Autodesk Inventor part; units mm, degrees
ref_plane "YZ Plane" through (0, 0, 0) normal (1, 0, 0) x (0, 1, 0)
ref_plane "XZ Plane" through (0, 0, 0) normal (0, 1, 0) x (-1, 0, 0)
ref_plane "XY Plane" through (0, 0, 0) normal (0, 0, 1) x (1, 0, 0)
sketch "Sketch1" plane through (0, 0, 0) normal (0, 0, 1) x (1, 0, 0)
  circle A0 centre (0, 0) radius 38.1
  line L0 (7.852, 0) -> (3.926, -6.8)
  line L1 (3.926, -6.8) -> (-3.926, -6.8)
  line L2 (-3.926, -6.8) -> (-7.852, 0)
  line L3 (-7.852, 0) -> (-3.926, 6.8)
  line L4 (-3.926, 6.8) -> (3.926, 6.8)
  line L5 (3.926, 6.8) -> (7.852, 0)
  circle A1 centre (0, 0) radius 31.75 construction
  circle A2 centre (0, 31.75) radius 2.413
  circle A3 centre (-15.875, 27.4963) radius 2.413
  circle A4 centre (-27.4963, 15.875) radius 2.413
  circle A5 centre (-31.75, 0) radius 2.413
  circle A6 centre (-27.4963, -15.875) radius 2.413
  circle A7 centre (-15.875, -27.4963) radius 2.413
  circle A8 centre (0, -31.75) radius 2.413
  circle A9 centre (15.875, -27.4963) radius 2.413
  circle A10 centre (27.4963, -15.875) radius 2.413
  circle A11 centre (31.75, 0) radius 2.413
  circle A12 centre (27.4963, 15.875) radius 2.413
  circle A13 centre (15.875, 27.4963) radius 2.413
  line L6 (-9.525, 25.4) -> (-3.9688, 13.15)
  line L7 (-3.9688, 13.15) -> (3.9688, 13.15)
  line L8 (3.9688, 13.15) -> (9.525, 25.4)
  line L9 (9.525, 25.4) -> (-9.525, 25.4)
  line L10 (0, -53.34) -> (0, 53.34) construction
  circle A14 centre (0, 0) radius 25.4 construction
  line L11 (0, 29.337) -> (0, 25.4)
  line L12 (0, 38.1) -> (0, 25.4)
  dimension "d0" = 76.2
  dimension "d2" = 63.5
  dimension "d3" = 4.826
  dimension "d1" = 13.6
  dimension "d6" = 360
  dimension "d16" = 6.35
  dimension "d18" = 7.9375
  dimension "d19" = 19.05
  dimension "d20" = 12.7
extrude "Extrusion1" add sketch "Sketch1" along normal blind 3.175 contours L9 L8 L7 L6 | A0
extrude "Extrusion2" cut sketch "Sketch1" along normal blind 3.175 contours L9 L8 L7 L6
fillet "Fillet1" radius 3.175 4 edges at (-9.525, 25.4, 1.5875) (9.525, 25.4, 1.5875) (-3.9688, 13.15, 1.5875) (3.9688, 13.15, 1.5875)
pattern_circular "Circular Pattern1" count 6 over 360 about axis through (0, 0, 0) along (0, 0, 1) of "Extrusion2", "Fillet1"
properties part number "ThickWheelPlate_v83DPrintable" material "Steel, Alloy"
The listing builds one solid part. Answer for the finished solid, in the listing's coordinates (mm). Round coordinates to 2 decimals unless told otherwise and drop trailing zeros. Order: outer loops, then holes, each group sorted by start corner. A loop starts at its lowest first (then second) coordinate and runs counter-clockwise, first axis right, second up. Notation, with made-up numbers: M 13.25,53 L 44.25,53 A20 cw 44.25,86 Z; hole C 89,-26.5 d9. An arc over 180 degrees is marked long. Answer in a Markdown table with one row per item. Add a question column.
1) The part is cut by section A-A on x = 0. Determine the outline of the cut face in (y, z) (3 decimals).
2) The part is cut by section D-D on y = -1. Determine the outline of the cut face in (x, z) (3 decimals).
3) The part is cut by section B-B on y = 31.75. Determine the outline of the cut face in (x, z) (3 decimals), plus the area to 3 significant figures.
4) Consider line 1 along Y through (x, z) = (0, 0.7); line 2 along Y through (x, z) = (-1.5, 0.85); line 3 along Y through (x, z) = (15, 1.2). Determine where each line is inside the solid, lowest interval first. Write a range as from..to.
5) Determine the mould class of faces 1 (the face through (-29.448, -0.725, 1.565)), 2 (the face through (-30.235, 23.183, 1.565)), 3 (the face through (13.671, -3.662, 1.61)) for opening direction Y: pulls with the +Y half, pulls with the -Y half, needs draft (parallel to the pull), parting line crosses it, or undercut.
6) Flat-ended cylindrical pins translate along their axes: pin 1 Ø1.6 at (x, z) = (-0.5, 1.5) entering from +Y; pin 2 Ø1.5 at (y, z) = (-8, 1) entering from +X. Find the tip coordinate at first contact, or state that the pin passes through.
Findings below:
| question | item | result |
|---|---|---|
| 1 | outline | M -38.1,0 L -34.163,0 L -34.163,3.175 L -38.1,3.175 Z; M -29.337,0 L -25.4,0 L -25.4,3.175 L -29.337,3.175 Z; M -13.15,0 L -6.8,0 L -6.8,3.175 L -13.15,3.175 Z; M 6.8,0 L 13.15,0 L 13.15,3.175 L 6.8,3.175 Z; M 25.4,0 L 29.337,0 L 29.337,3.175 L 25.4,3.175 Z; M 34.163,0 L 38.1,0 L 38.1,3.175 L 34.163,3.175 Z |
| 2 | outline | M -38.087,0 L -33.946,0 L -33.946,3.175 L -38.087,3.175 Z; M -29.554,0 L -7.275,0 L -7.275,3.175 L -29.554,3.175 Z; M 7.275,0 L 29.554,0 L 29.554,3.175 L 7.275,3.175 Z; M 33.946,0 L 38.087,0 L 38.087,3.175 L 33.946,3.175 Z |
| 3 | outline | M -21.061,0 L -2.413,0 L -2.413,3.175 L -21.061,3.175 Z; M 2.413,0 L 21.061,0 L 21.061,3.175 L 2.413,3.175 Z |
| 3 | area | 118 mm² |
| 4 | line 1 | y = -38.1..-34.16, -29.34..-25.4, -13.15..-6.8, 6.8..13.15, 25.4..29.34, 34.16..38.1 |
| 4 | line 2 | y = -38.07..-33.64, -29.86..-25.4, -13.15..-6.8, 6.8..13.15, 25.4..29.86, 33.64..38.07 |
| 4 | line 3 | y = -35.02..-29.75, -25.25..-17.6, -3.32..3.32, 17.6..25.25, 29.75..35.02 |
| 5 | face 1 | undercut |
| 5 | face 2 | parting line crosses it |
| 5 | face 3 | undercut |
| 6 | pin 1 | stops at y = 38.1 |
| 6 | pin 2 | stops at x = 37.4 |
